Here's how the part is built. I have some questions about the finished solid (model axes, mm). Give positions to 0.01 mm unless a question says otherwise; leave off trailing zeros. Write each loop counter-clockwise with the first axis right and the second up, starting at its lowest first coordinate (ties: lowest second). Pieces come first, ordered by that corner, then holes. Notation, with made-up numbers: (88.5, 2) - (96.5, 2) arc R18 cw to (96.5, 37) - close; hole circle Ø6 at (-3.75, 83.25). An arc over 180 degrees is marked (long way). Write each question's results on one line, items separated by ' | '. Start each with the question number.
Item 1: Suppose I cut it at D-D on z = -5.75. List the corners of the cut face in (x, y) for me.
Item 2: We'd pull the mould along Y, two halves only. Please class faces 1 (the cylindrical face through (-0.521, 18.966, 0.147)), 2 (the flat face through (0, 100, 0)), 3 (the flat face through (-10.5, 49, 5)): +Y half, -Y half, draft (parallel to the pull), parting line (faces both ways), or undercut.
Item 3: Please list where these lines run through material, in increasing order: line 1 along Y through (x, z) = (0, 4.5); line 2 along Y through (x, z) = (-6, 0); line 3 along Y through (x, z) = (-2.75, -8).
Item 4: Suppose I cut it at C-C on y = 15. List the corners of the cut face in (x, z) for me.
Item 5: Suppose I cut it at B-B on x = 0. List the corners of the cut face in (y, z) for me, then the cut area to 3 significant figures.
Item 6: Suppose I cut it at A-A on z = 0. List the corners of the cut face in (x, y) for me, then the cut area to 3 significant figures.
```python
from build123d import *

# Parameters (mm, degrees)
SKETCH1_W           = 21
SKETCH1_H           = 21
BOSS_EXTRUDE1_DEPTH = 100
SKETCH2_R           = 4
CUT_EXTRUDE1_DEPTH  = 103.719277645
SKETCH4_R           = 4
CUT_EXTRUDE2_DEPTH  = 103.719277645


with BuildPart() as part:
    # Sketch1 → Boss-Extrude1 (new body)
    with BuildSketch(Plane(origin=(0, 0, 0), x_dir=(1, 0, 0), z_dir=(0, 1, 0))):
        Rectangle(SKETCH1_W, SKETCH1_H)
    extrude(amount=BOSS_EXTRUDE1_DEPTH)

    # Sketch2 → Cut-Extrude1 (cut, through all)
    with BuildSketch(Plane.XY.offset(10.5)):
        with Locations((0, 85)):
            Circle(SKETCH2_R)
        with Locations((0, 15)):
            Circle(SKETCH2_R)
    extrude(amount=-CUT_EXTRUDE1_DEPTH, mode=Mode.SUBTRACT)

    # Sketch4 → Cut-Extrude2 (cut, through all)
    with BuildSketch(Plane(origin=(10.5, 0, 0), x_dir=(0, 0, -1), z_dir=(1, 0, 0))):
        with Locations((0, 50)):
            Circle(SKETCH4_R)
    extrude(amount=-CUT_EXTRUDE2_DEPTH, mode=Mode.SUBTRACT)


solid = part.part
```
Checked values:
1) outline: (-10.5, 0) - (10.5, 0) - (10.5, 100) - (-10.5, 100) - close; hole circle Ø8 at (0, 15); hole circle Ø8 at (0, 85)
2) face 1: undercut | face 2: +Y half | face 3: draft
3) line 1: y = 0 to 11, 19 to 81, 89 to 100 | line 2: y = 0 to 46, 54 to 100 | line 3: y = 0 to 12.1, 17.9 to 82.1, 87.9 to 100
4) outline: (-10.5, -10.5) - (-4, -10.5) - (-4, 10.5) - (-10.5, 10.5) - close; (4, -10.5) - (10.5, -10.5) - (10.5, 10.5) - (4, 10.5) - close
5) outline: (0, -10.5) - (11, -10.5) - (11, 10.5) - (0, 10.5) - close; (19, -10.5) - (81, -10.5) - (81, 10.5) - (19, 10.5) - close; (89, -10.5) - (100, -10.5) - (100, 10.5) - (89, 10.5) - close; hole circle Ø8 at (50, 0) | area: 1,710 mm^2
6) outline: (-10.5, 0) - (10.5, 0) - (10.5, 46) - (-10.5, 46) - close; (-10.5, 54) - (10.5, 54) - (10.5, 100) - (-10.5, 100) - close; hole circle Ø8 at (0, 15); hole circle Ø8 at (0, 85) | area: 1,830 mm^2
